from build123d import *

# Parameters (mm, degrees)
SKETCH1_R           = 2.2
BOSS_EXTRUDE1_DEPTH = 6.2
CUT_EXTRUDE1_DEPTH  = 1


with BuildPart() as part:
    # Sketch1 → Boss-Extrude1 (new body)
    with BuildSketch(Plane(origin=(0, 0, 0), x_dir=(-1, 0, 0), z_dir=(0, 0, 1))):
        Polygon((-144.298520867, 82.267611076), (-149.806405315, 88.04360735), (-167.861763168, 106.127941253), (-173.899609442, 100.09976926), (-149.860209976, 76.964086023), align=None)
        with Locations((-149.935011138, 82.733649845)):
            Circle(SKETCH1_R, mode=Mode.SUBTRACT)
        with Locations((-168.087755201, 100.095717423)):
            Circle(SKETCH1_R, mode=Mode.SUBTRACT)
    extrude(amount=BOSS_EXTRUDE1_DEPTH)

    # Sketch2 → Cut-Extrude1 (cut)
    with BuildSketch(Plane.XY.offset(6.2)):
        with BuildLine():
            Line((156.351932178, -87.573874819), (156.351932178, -87.899515844))
            Line((156.351932178, -87.899515844), (155.271974245, -87.899515844))
            Line((155.271974245, -87.899515844), (155.100885503, -88.73460699))
            add(Edge.make_bspline(
                [(155.100885503, -88.73460699), (155.134500475, -88.725326672), (155.199624166, -88.707347524), (155.295744897, -88.687385146), (155.386996396, -88.675351494), (155.446210482, -88.673708376), (155.474863868, -88.67291328)],
                knots=[0, 0, 0, 0, 0.000104595, 0.000202637, 0.000294305, 0.000380252, 0.000380252, 0.000380252, 0.000380252], degree=3))
            add(Edge.make_bspline(
                [(155.474863868, -88.67291328), (155.510318404, -88.673680665), (155.580030878, -88.675189535), (155.682029066, -88.689678284), (155.779395334, -88.712483778), (155.871926055, -88.744343108), (155.959792412, -88.785082652), (156.042185985, -88.835973312), (156.120343521, -88.895421405), (156.192862874, -88.963770095), (156.258652782, -89.038991847), (156.316497644, -89.119870773), (156.365630851, -89.205620866), (156.405146679, -89.297061419), (156.436701039, -89.393181508), (156.457703206, -89.494992493), (156.471688363, -89.601534717), (156.473250814, -89.674382434), (156.474047562, -89.711530067)],
                knots=[0, 0, 0, 0, 0.000106308, 0.000209029, 0.000308378, 0.000405929, 0.000502102, 0.000598312, 0.00069588, 0.000796219, 0.000896736, 0.000995218, 0.001094066, 0.001192613, 0.001293582, 0.001396995, 0.001504047, 0.001615439, 0.001615439, 0.001615439, 0.001615439], degree=3))
            add(Edge.make_bspline(
                [(156.474047562, -89.711530067), (156.473444244, -89.737403796), (156.472245761, -89.788801592), (156.466151042, -89.865132402), (156.4544165, -89.939847258), (156.438661493, -90.012956071), (156.418212299, -90.08432043), (156.393457229, -90.154144601), (156.363162261, -90.221993995), (156.329932371, -90.288510603), (156.292515923, -90.352190677), (156.250988277, -90.411743687), (156.207113867, -90.468062999), (156.159904896, -90.5205446), (156.108922565, -90.568843623), (156.054784309, -90.613246707), (155.997922128, -90.654504771), (155.937456301, -90.690943062), (155.874734192, -90.724473744), (155.808850023, -90.751981524), (155.741303531, -90.776574646), (155.671122536, -90.796177575), (155.598466006, -90.811537821), (155.523214174, -90.821970508), (155.445761709, -90.829569134), (155.393260805, -90.8300448), (155.366740872, -90.830285075)],
                knots=[0, 0, 0, 0, 7.7636e-05, 0.000154223, 0.000229512, 0.000304362, 0.000378447, 0.000452077, 0.000526407, 0.000601214, 0.00067506, 0.000747747, 0.00081887, 0.000889121, 0.000959302, 0.001029336, 0.001099058, 0.00116985, 0.001240974, 0.00131221, 0.00138383, 0.001456517, 0.001530612, 0.001606437, 0.001684346, 0.001763871, 0.001763871, 0.001763871, 0.001763871], degree=3))
            add(Edge.make_bspline(
                [(155.366740872, -90.830285075), (155.335105008, -90.829658386), (155.272865183, -90.82842545), (155.181678668, -90.815527253), (155.093944705, -90.797054272), (155.010369541, -90.769262798), (154.930204181, -90.734440038), (154.854527858, -90.69042894), (154.781406904, -90.640555039), (154.713813842, -90.58169929), (154.651079368, -90.517368635), (154.594921321, -90.447557061), (154.54490729, -90.373416781), (154.501838191, -90.294587742), (154.4651007, -90.211277074), (154.436239961, -90.123172638), (154.412946025, -90.030734777), (154.403091351, -89.967095521), (154.398086024, -89.934772255)],
                knots=[0, 0, 0, 0, 9.4843e-05, 0.000186593, 0.000275792, 0.000363484, 0.000450342, 0.000537514, 0.000625728, 0.000715478, 0.000805885, 0.000894984, 0.00098389, 0.001073836, 0.001164117, 0.001256635, 0.001351658, 0.001449737, 0.001449737, 0.001449737, 0.001449737], degree=3))
            Line((154.398086024, -89.934772255), (154.683021921, -89.934772255))
            add(Edge.make_bspline(
                [(154.683021921, -89.934772255), (154.690032827, -89.965049465), (154.703508177, -90.023243945), (154.733086249, -90.105005947), (154.769250293, -90.177866957), (154.812252809, -90.242790794), (154.863551765, -90.29940467), (154.922089176, -90.34985729), (154.987718896, -90.3953733), (155.06064704, -90.433312525), (155.137584619, -90.46566918), (155.21810916, -90.48721536), (155.300028103, -90.502365456), (155.35543491, -90.503881982), (155.38327733, -90.50464405)],
                knots=[0, 0, 0, 0, 9.3172e-05, 0.000179081, 0.000260145, 0.000336703, 0.000411917, 0.000488562, 0.000568128, 0.000650923, 0.00073478, 0.000817953, 0.000900557, 0.000983994, 0.000983994, 0.000983994, 0.000983994], degree=3))
            add(Edge.make_bspline(
                [(155.38327733, -90.50464405), (155.410453919, -90.503899487), (155.463964845, -90.502433437), (155.542715174, -90.491149476), (155.618745424, -90.473770822), (155.691305384, -90.447763167), (155.76166478, -90.41615403), (155.828043843, -90.375591068), (155.892362882, -90.32890948), (155.952622689, -90.275427394), (156.007812761, -90.2164906), (156.056577242, -90.153464679), (156.097196299, -90.086230111), (156.131426526, -90.015950894), (156.157419162, -89.941856774), (156.175962052, -89.864294994), (156.186850541, -89.783073976), (156.188348397, -89.727675388), (156.189111665, -89.699445732)],
                knots=[0, 0, 0, 0, 8.15e-05, 0.000160473, 0.000238226, 0.000315066, 0.000391338, 0.000469218, 0.000547964, 0.000629516, 0.000710512, 0.000789892, 0.000868102, 0.000945761, 0.001024012, 0.00110315, 0.001184644, 0.001269321, 0.001269321, 0.001269321, 0.001269321], degree=3))
            add(Edge.make_bspline(
                [(156.189111665, -89.699445732), (156.18851433, -89.673977015), (156.187345132, -89.624125624), (156.1777924, -89.551192058), (156.16117629, -89.482182941), (156.138113198, -89.416765029), (156.108831074, -89.354876621), (156.073047633, -89.296453844), (156.030091336, -89.242266724), (155.981022266, -89.192289908), (155.927266758, -89.146166343), (155.867899934, -89.106847064), (155.804164143, -89.073769082), (155.736827292, -89.045223112), (155.664287706, -89.024721007), (155.587981903, -89.009328711), (155.50708589, -89.000424775), (155.451776766, -88.999189348), (155.423346441, -88.998554306)],
                knots=[0, 0, 0, 0, 7.6388e-05, 0.000149519, 0.000220172, 0.000288967, 0.000357247, 0.000425206, 0.000494043, 0.000564207, 0.000635056, 0.000706145, 0.000777268, 0.000850264, 0.000925136, 0.001002969, 0.001083601, 0.001168886, 0.001168886, 0.001168886, 0.001168886], degree=3))
            add(Edge.make_bspline(
                [(155.423346441, -88.998554306), (155.398736627, -88.999080985), (155.347923604, -89.000168444), (155.269979326, -89.008175337), (155.188071834, -89.021092412), (155.102515113, -89.038859936), (155.013052224, -89.062110984), (154.91987196, -89.089973424), (154.822778404, -89.123285523), (154.757357326, -89.148442603), (154.72372705, -89.161374819)],
                knots=[0, 0, 0, 0, 7.3822e-05, 0.000152423, 0.000234822, 0.000322511, 0.00041445, 0.000512043, 0.000614219, 0.000722306, 0.000722306, 0.000722306, 0.000722306], degree=3))
            Line((154.72372705, -89.161374819), (155.049368075, -87.573874819))
            Line((155.049368075, -87.573874819), (156.351932178, -87.573874819))
        make_face()
        Polygon((158.532836625, -87.492464562), (158.590714229, -87.492464562), (158.590714229, -89.690541485), (158.957060383, -89.690541485), (158.957060383, -90.016182511), (158.590714229, -90.016182511), (158.590714229, -90.748874819), (158.305778332, -90.748874819), (158.305778332, -90.016182511), (156.799688588, -90.016182511), align=None)
        Polygon((158.305778332, -89.690541485), (158.305778332, -88.311655268), (157.359384101, -89.690541485), align=None, mode=Mode.SUBTRACT)
    extrude(amount=-CUT_EXTRUDE1_DEPTH, mode=Mode.SUBTRACT)


solid = part.part
Part model, mm, in its own coordinate system. A direction names the side the tool comes from. Give positions to 0.01 mm unless a question says otherwise; leave off trailing zeros. Order: outer loops, then holes, each group sorted by start corner. A loop starts at its lowest first (then second) coordinate and runs counter-clockwise, first axis right, second up. Notation, with made-up numbers: (81.5, 34) - (101.5, 34) arc R14 cw to (101.5, 43) - close; hole circle Ø7 at (21.25, 42.25). An arc over 180 degrees is marked (long way). One line per question, with ' | ' between items.
1. Band-saw the part on B-B on y = -84.5. List the corners of the cut face in (x, z), then the cut area to 3 significant figures.
Filled in:
outline: (146.43, 0) - (148.62, 0) - (148.62, 6.2) - (146.43, 6.2) - close; (151.25, 0) - (157.69, 0) - (157.69, 6.2) - (151.25, 6.2) - close | area: 53.6 mm²
2. Band-saw the part on C-C on z = 5.75. Give the number of separate pieces and of enclosed holes in the cut face, then the cut area to 3 significant figures.
Filled in:
separate pieces: 2 | enclosed holes: 4 | area: 239 mm²
3. Band-saw the part on A-A on x = 167.5. List the corners of the cut face in (y, z).
Filled in:
outline: (-105.77, 0) - (-102.22, 0) - (-102.22, 6.2) - (-105.77, 6.2) - close; (-97.98, 0) - (-93.94, 0) - (-93.94, 6.2) - (-97.98, 6.2) - close
4. Band-saw the part on D-D on z = 2.5. List the corners of the cut face in (x, y), then the cut area to 3 significant figures.
Filled in:
outline: (144.3, -82.27) - (149.81, -88.04) - (167.86, -106.13) - (173.9, -100.1) - (149.86, -76.96) - close; hole circle Ø4.4 at (149.94, -82.73); hole circle Ø4.4 at (168.09, -100.1) | area: 243 mm²
5. Drop flat-ended pins along their axis: P1, Ø1, axis at x = 169, z = 5, coming from the +Y side; P2, Ø3, axis at y = -82.5, z = 2, coming from the -X side; P3, Ø0.8, axis at y = -89, z = 6, coming from the -X side. Give the stop position or say it passes through.
Filled in:
P1: y = -94.9 | P2: x = 144.3 | P3: x = 150.36
6. Drill centre lines: probe 1 along X at (y, z) = (-101, 3); probe 2 along Y at (x, z) = (158, 5.5); probe 3 along X at (y, z) = (-83.25, 2). Where is each one in solid material? Low to high.
Filled in:
probe 1: 162.74 to 166.08, 170.09 to 173 | probe 2: -96.25 to -90.02, -89.69 to -88.76, -88.27 to -84.8 | probe 3: 145.24 to 147.8, 152.07 to 156.39
7. Which spindle directions (+Z, -Z, +X, -X, +Y, -Y) get a long thin tool onto all of the face, cutting with end or side? Do faces 1 (the face through (158.71, -96.96, 3.06)), 2 (the face through (156, -87.9, 6)). Say none if no direction does.
Filled in:
face 1: +Z, -Z, -X, -Y | face 2: +Z
